```python
from build123d import *

# Parameters (mm, degrees)
F1_DEPTH = 63.5
F2_DEPTH = 7.9375
F0_W     = 25.4
F0_H     = 19.05
F3_DEPTH = 25.4


with BuildPart() as f1:
    # F0 (on Front) → F1 (new body, symmetric)
    with BuildSketch(Plane.XZ):
        Polygon((-41.275, 9.525), (-41.275, -9.525), (41.275, -9.525), (41.275, 9.525), (22.225, 9.525), align=None)
    extrude(amount=F1_DEPTH, both=True)

    # F0 (on Front) → F2 (join, symmetric)
    with BuildSketch(Plane.XZ):
        with BuildLine():
            add(Edge.make_bspline(
                [(-41.275, 9.525), (-4.041549, 19.120571), (15.072903, 58.732133), (53.711712, 61.755542)],
                knots=[0, 0, 0, 0, 108.338644, 108.338644, 108.338644, 108.338644], degree=3))
            Line((-41.275, 9.525), (22.225, 9.525))
            Line((22.225, 9.525), (22.225, 27.0002))
            ThreePointArc((22.225, 27.0002), (31.267208, 50.448797), (53.711712, 61.755542))
        make_face()
    extrude(amount=F2_DEPTH, both=True)

    # F0 (on Front) → F3 (join, symmetric)
    with BuildSketch(Plane.XZ):
        with BuildLine():
            Line((22.225, 9.525), (41.275, 9.525))
            Line((41.275, 9.525), (41.275, 27.0002))
            ThreePointArc((41.275, 27.0002), (45.92468, 38.22552), (57.15, 42.8752))
            Line((57.15, 42.8752), (60.325, 42.8752))
            Line((60.325, 42.8752), (60.325, 61.9252))
            Line((60.325, 61.9252), (57.15, 61.9252))
            add(Edge.make_bspline(
                [(53.711712, 61.755542), (54.840822, 61.843893), (55.986605, 61.900999), (57.15, 61.9252)],
                knots=[108.338644, 108.338644, 108.338644, 108.338644, 111.504536, 111.504536, 111.504536, 111.504536], degree=3))
            ThreePointArc((53.711712, 61.755542), (31.267208, 50.448797), (22.225, 27.0002))
            Line((22.225, 27.0002), (22.225, 9.525))
        make_face()
        with Locations((73.025, 52.4002)):
            Rectangle(F0_W, F0_H)
    extrude(amount=F3_DEPTH, both=True)

    # F0 (on Front) → F4 (revolve)
    with BuildSketch(Plane.XZ):
        Polygon((85.725, 66.675), (85.725, 61.9252), (85.725, 42.8752), (85.725, 38.1), (111.125, 38.1), (111.125, 66.675), align=None)
    revolve(axis=Axis((85.725, 0, 52.4002), (0, 0, -1)))


solid = f1.part
```
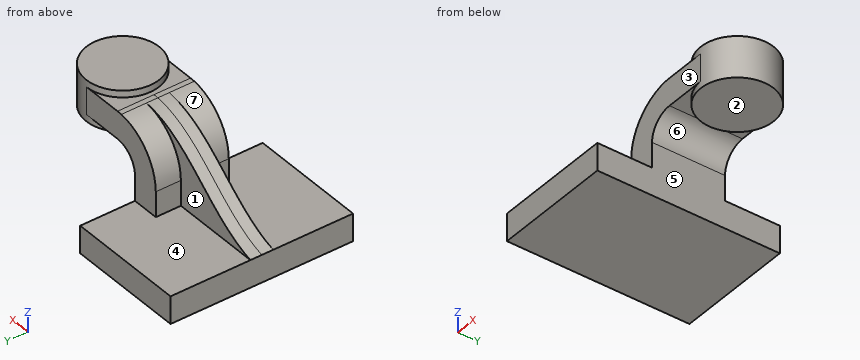
Check sheet for the modelled part. Datum: model origin and axes. Units: mm. Face numbers are marked on the shaded views. A direction names the side the tool comes from. Coordinates: 2 decimals unless noted, no trailing zeros. Order: outer loops, then holes, each group sorted by start corner. A loop starts at its lowest first (then second) coordinate and runs counter-clockwise, first axis right, second up. Notation, with made-up numbers: M 18,86 L 69,86 A25 cw 69,107 Z; hole C 55.25,20 d2. An arc over 180 degrees is marked long. Write each question's results on one line, items separated by ' | '. Start each with the question number.
1. Access from +Z, -Z, +X, -X, +Y, -Y to the whole of each face (thin tool, end or side, straight path). Record for the marked faces 1, 2 and 3.
2. Go/stop test with flat-tipped pins: P1, Ø18.5, axis at y = 17, z = 8, coming from the +X side (3 decimals); P2, Ø1.5, axis at x = 94.5, y = -5, coming from the -Z side; P3, Ø19, axis at y = -19.5, z = 22.5, coming from the -X side (3 decimals). Record where each tip stops, or that it passes through.
3. Cross-section at B-B on z = 2.5. Record the cut outline in (x, y) (3 decimals), and give its area (3 significant figures).
4. Mould release check, pull along X, two halves, no side actions. Record for the marked faces 4, 5, 6 and 7: +X half, -X half, draft (parallel to the pull), parting line (faces both ways), or undercut.
5. Cross-section at A-A on y = 37. Record the cut outline in (x, z) (3 decimals).
6. Material ranges on probe 1 along X at (y, z) = (-36, 1) (3 decimals); probe 2 along X at (y, z) = (-18, 15) (3 decimals); probe 3 along Z at (x, y) = (66, 11) (3 decimals), recorded low to high.
Checks:
1) face 1: +Z, -X, +Y | face 2: -Z, +X, +Y, -Y | face 3: +Z, +X, -X, -Y
2) P1: stops at x = 41.275 | P2: stops at z = 38.1 | P3: stops at x = 22.225
3) outline: M -41.275,-63.5 L 41.275,-63.5 L 41.275,63.5 L -41.275,63.5 Z | area: 10,500 mm²
4) face 4: draft | face 5: +X half | face 6: undercut | face 7: -X half
5) outline: M -41.275,-9.525 L 41.275,-9.525 L 41.275,9.525 L -41.275,9.525 Z
6) probe 1: x = -41.275 to 41.275 | probe 2: x = 22.225 to 41.275 | probe 3: z = 38.1 to 66.675
